The listing builds one solid part. Answer for the finished solid, in the listing's coordinates (mm). Face numbers are marked on the shaded views. A direction names the side the tool comes from. Round coordinates to 2 decimals unless told otherwise and drop trailing zeros. Loops run counter-clockwise (first coordinate to the right, second up) from the corner with the lowest first, then second, coordinate; pieces in that order, holes last. Notation, with made-up numbers: (11, 70.25) - (39, 70.25) arc R18 ccw to (39, 91.25) - close; hole circle Ø4 at (46, 30.25). An arc over 180 degrees is marked (long way). One line per question, with ' | ' between items. Start each with the question number.
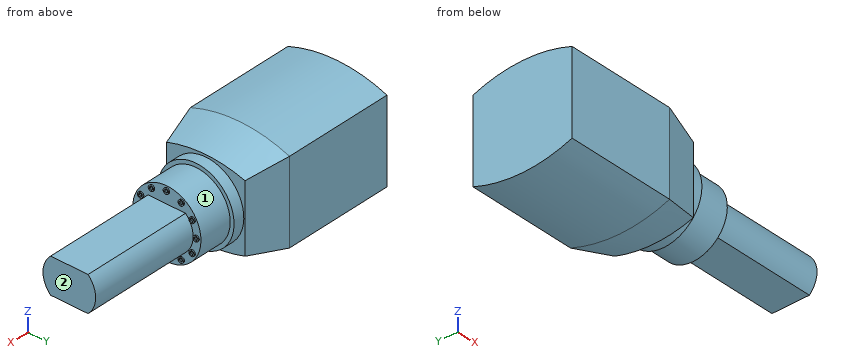
Autodesk Fusion 360 part; units mm, degrees
sketch "Sketch1" plane through (0, 0, 0) normal (1, 0, 0) x (0, 0, -1)
  line L0 (0, 0) -> (0, 45)
  line L1 (0, 0) -> (0, -45)
  line L2 (0, 45) -> (37.5, 45)
  line L3 (0, 45) -> (-37.5, 45)
  line L4 (0, -45) -> (37.5, -45)
  line L5 (0, -45) -> (-37.5, -45)
  arc A0 (-37.5, 45) -> (-37.5, -45) centre (79.119, 0) ccw
  arc A1 (37.5, -45) -> (37.5, 45) centre (-79.119, 0) ccw
  dimension "d1" = 45
  dimension "d2" = 45
  dimension "d3" = 37.5
  dimension "d4" = 37.5
  dimension "d5" = 37.5
  dimension "d6" = 37.5
  dimension "d8" = 125
extrude "Extrude1" add sketch "Sketch1" along normal blind 100
extrude "Extrude2" add 1 faces at (100, -15.2642, -14.2806) along direction (1, 0, 0) blind 35 draft -15
sketch "Sketch2" plane through (135, 0, 0) normal (1, 0, 0) x (0, 0, -1)
  line L0 (-30.8786, -35.6218) -> (30.8786, -35.6218)
  arc A0 (30.8786, -35.6218) -> (30.8786, 35.6218) centre (-79.119, 0) ccw
  line L1 (30.8786, 35.6218) -> (-30.8786, 35.6218)
  arc A1 (-30.8786, 35.6218) -> (-30.8786, -35.6218) centre (79.119, 0) ccw
  circle A2 centre (0, 0) radius 34.5
  dimension "d13" = 69
extrude "Extrude3" add sketch "Sketch2" along normal blind 10 contours A2
sketch "Sketch3" plane through (145, 0, 0) normal (1, 0, 0) x (0, 0, -1)
  circle A0 centre (0, 0) radius 34.5
  circle A1 centre (0, 0) radius 31
  dimension "d16" = 62
extrude "Extrude4" add sketch "Sketch3" along normal blind 30 contours A1
sketch "Sketch4" plane through (175, 0, 0) normal (1, 0, 0) x (0, 0, -1)
  circle A0 centre (0, 0) radius 31
  line L0 (0, 0) -> (27, 0)
  circle A1 centre (27, 0) radius 2.5
  circle A2 centre (27, 0) radius 1.5
  dimension "d19" = 27
  dimension "d20" = 5
  dimension "d21" = -1
extrude "Extrude5" add sketch "Sketch4" along normal blind 1 contours A1
pattern_circular "C-Pattern1" count 12 over 360 about axis through (175, 0, 0) along (1, 0, 0) of "Extrude5"
sketch "Sketch5" plane through (175, 0, 0) normal (1, 0, 0) x (0, 0, -1)
  circle A0 centre (27, 0) radius 2.5
  circle A1 centre (0, 0) radius 31
  circle A2 centre (23.3827, 13.5) radius 2.5
  circle A3 centre (13.5, 23.3827) radius 2.5
  circle A4 centre (0, 27) radius 2.5
  circle A5 centre (-13.5, 23.3827) radius 2.5
  circle A6 centre (-23.3827, 13.5) radius 2.5
  circle A7 centre (-27, 0) radius 2.5
  circle A8 centre (-23.3827, -13.5) radius 2.5
  circle A9 centre (-13.5, -23.3827) radius 2.5
  circle A10 centre (0, -27) radius 2.5
  circle A11 centre (13.5, -23.3827) radius 2.5
  circle A12 centre (23.3827, -13.5) radius 2.5
  line L0 (0, 0) -> (16, 0)
  line L1 (16, 0) -> (16, 17)
  line L2 (16, 0) -> (16, -17)
  line L3 (0, 0) -> (0, -8.0593)
  line L4 (-16, 0) -> (-16, 17)
  line L5 (-16, 0) -> (-16, -17)
  arc A13 (16, 17) -> (-16, 17) centre (0, 1.9003) ccw
  arc A14 (-16, -17) -> (16, -17) centre (0, -1.9003) ccw
  dimension "d26" = 16
  dimension "d27" = 17
  dimension "d28" = 17
  dimension "d29" = 22
extrude "Extrude6" add sketch "Sketch5" along normal blind 100 contours L1 L2 L4 L5 A13 A14
(1) Find section A-A on x = 180.5. Write down the section's boundary in (y, z), plus the area to 3 significant figures.
(2) A tool of negligible diameter and unlimited length cuts with its end or side. For the marked faces 1 and 2, from which of +Z, -Z, +X, -X, +Y, -Y can it reach the whole face along a straight path? Write none if from no direction.
(3) Find section B-B on x = 107.5. Write down the section's boundary in (y, z).
(4) Consider L1, parallel to Y at x = 138, z = -0.5; L2, parallel to X at y = 28.5, z = -21; L3, parallel to Z at x = 60, y = 0.5. Determine where each line is inside the solid, lowest interval first.
(5) Each of these flat-tipped pins is pushed along its axis until it touches: P1, Ø1.5, axis at y = -26.5, z = 0, coming from the +X side; P2, Ø5, axis at y = 27, z = 0, coming from the +X side; P3, Ø2, axis at x = 96, y = 10, coming from the +Z side; P4, Ø1.8, axis at y = -27, z = 0, coming from the -X side. Where does it stop, or does it pass through?
Answer below:
1) outline: (-17, -16) - (17, -16) arc R22 ccw to (17, 16) - (-17, 16) arc R22 ccw to start | area: 1,390 mm2
2) face 1: +X | face 2: +Z, -Z, +X, +Y, -Y
3) outline: (-42.99, -36.11) arc R122.99 ccw to (42.99, -36.11) - (42.99, 36.11) arc R122.99 ccw to (-42.99, 36.11) - close
4) L1: -34.5 to 34.5 | L2: 0 to 135 | L3: -45.88 to 45.88
5) P1: x = 175 | P2: x = 176 | P3: z = 45.56 | P4: x = 0
